Verification items for this drawing (mm, ordinates from the low corner). Round coordinates to 2 decimals unless told otherwise and drop trailing zeros. Loops run counter-clockwise (first coordinate to the right, second up) from the corner with the lowest first, then second, coordinate; pieces in that order, holes last. Notation, with made-up numbers: (59.25, 73) - (87.25, 73) arc R18 cw to (87.25, 86) - close; hole circle Ø2 at (44.25, 24.25). An arc over 180 degrees is marked (long way). Answer in a Markdown table with one row per item. Add a question column.
(1) Cross-section at A-A on z = 12.25. Enter the section's corners in (x, y), then the cut area to 3 significant figures.
(2) Gauge pin test, flat ends, axial feed: pin 1 (6 mm diameter, centred on y = 11, z = 3, fed in from +X) (1 decimal); pin 2 (5 mm diameter, centred on x = 10, y = 8.5, fed in from +Z). Record the tip position at first contact, or that the pin passes through.
(3) Thickness scan on line 1 along Z through (x, y) = (5.75, 5) (1 decimal); line 2 along Z through (x, y) = (3.75, 9); line 3 along Y through (x, z) = (8.25, 10.75). Record the ranges inside material, lowest first.
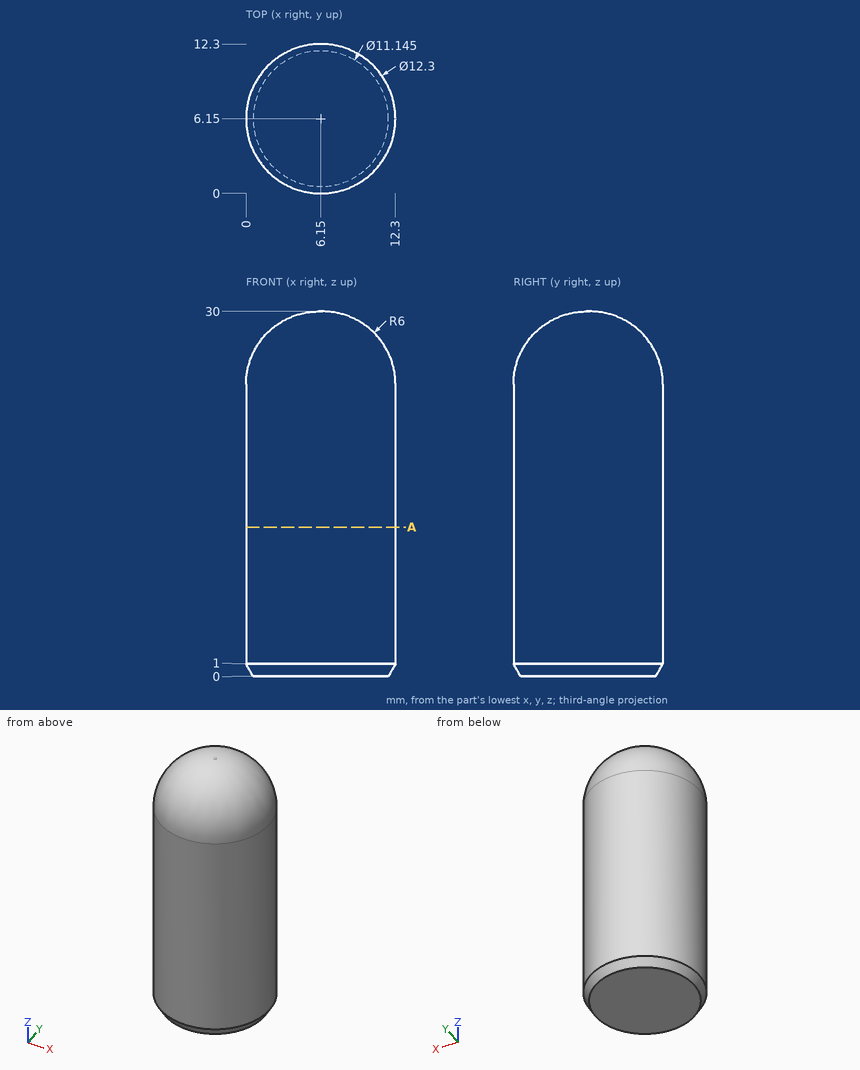
Answers:
| question | item | result |
|---|---|---|
| 1 | outline | circle Ø12.3 at (6.15, 6.15) |
| 1 | area | 119 mm^2 |
| 2 | pin 1 | stops at x = 12 |
| 2 | pin 2 | stops at z = 29.7 |
| 3 | line 1 | z = 0 to 29.9 |
| 3 | line 2 | z = 0 to 28.82 |
| 3 | line 3 | y = 0.37 to 11.93 |
